Design review of the part built by this model. Coordinates are the model's own, in mm. Face numbers are marked on the shaded views. Coordinates: 2 decimals unless noted, no trailing zeros. Loops run counter-clockwise (first coordinate to the right, second up) from the corner with the lowest first, then second, coordinate; pieces in that order, holes last. Notation, with made-up numbers: M -31.75,24 L 12.25,24 A16 cw 12.25,48 Z; hole C 34,-32 d11. An arc over 180 degrees is marked long. One line per item, written item: value.
```python
from build123d import *

# Parameters (mm, degrees)
SKETCH1_R           = 20
BOSS_EXTRUDE1_DEPTH = 50
SHELL3_T            = -2
CUT_EXTRUDE1_DEPTH  = 50


with BuildPart() as part:
    # Sketch1 → Boss-Extrude1 (new body)
    with BuildSketch(Plane(origin=(0, 0, 0), x_dir=(1, 0, 0), z_dir=(0, 1, 0))):
        with Locations(Location((0, 0, 0), (0, 0, 270))):
            Circle(SKETCH1_R)
    extrude(amount=BOSS_EXTRUDE1_DEPTH)

    # Shell3
    shell3_openings = [part.faces().sort_by_distance(p)[0] for p in [
        (0, 50, 0),
    ]]
    offset(amount=SHELL3_T, openings=shell3_openings, kind=Kind.INTERSECTION)

    # Sketch2 → Cut-Extrude1 (cut)
    with BuildSketch(Plane(origin=(0, 2, 0), x_dir=(1, 0, 0), z_dir=(0, 1, 0))):
        with BuildLine():
            Line((-1, -16.970562748), (-1, 16.970562748))
            ThreePointArc((-1, 16.970562748), (-17, 0), (-1, -16.970562748))
        make_face()
        with BuildLine():
            ThreePointArc((17, 0), (12.369316877, 11.66190379), (1, 16.970562748))
            Line((1, 16.970562748), (1, -16.970562748))
            ThreePointArc((1, -16.970562748), (12.369316877, -11.66190379), (17, 0))
        make_face()
    extrude(amount=-CUT_EXTRUDE1_DEPTH, mode=Mode.SUBTRACT)


solid = part.part
```
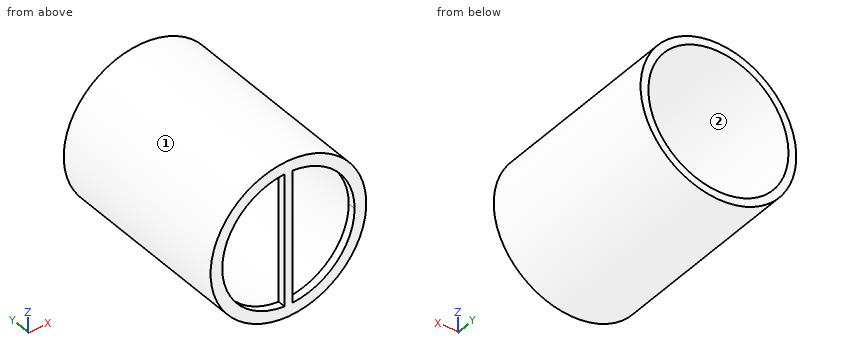
(1) We need section C-C on x = 0. State the section outline as (y, z) points.
Reply:
outline: M 0,-20 L 50,-20 L 50,-18 L 2,-18 L 2,18 L 50,18 L 50,20 L 0,20 Z
(2) We need section A-A on z = 1. State the section outline as (x, y) points, then the cut area to 3 significant figures.
Reply:
outline: M -19.97,0 L -16.97,0 L -16.97,2 L -17.97,2 L -17.97,50 L -19.97,50 Z; M -1,0 L 1,0 L 1,2 L -1,2 Z; M 16.97,0 L 19.97,0 L 19.97,50 L 17.97,50 L 17.97,2 L 16.97,2 Z
area: 208 mm2
(3) We need section B-B on x = 4.5. State the section outline as (y, z) points, then the cut area to 3 significant figures.
Reply:
outline: M 0,-19.49 L 50,-19.49 L 50,-17.43 L 2,-17.43 L 2,-16.39 L 0,-16.39 Z; M 0,16.39 L 2,16.39 L 2,17.43 L 50,17.43 L 50,19.49 L 0,19.49 Z
area: 210 mm2
(4) To check wall thickness, follow line 1 along X through (y, z) = (30, 0); line 2 along Z through (x, y) = (0.5, 15); line 3 along Z through (x, y) = (5.5, 23.5). State the ranges of each line that lie inside material, in increasing order. Write a range as [from, to].
Reply:
line 1: x = [-20, -18], [18, 20]
line 2: z = [-19.99, -17.99], [17.99, 19.99]
line 3: z = [-19.23, -17.14], [17.14, 19.23]
(5) Insertion check: pin 1 (4 mm diameter, centred on y = 24.5, z = -13.5, fed in from +X); pin 2 (1.6 mm diameter, centred on y = 1, z = -7.5, fed in from -X); pin 3 (1.5 mm diameter, centred on y = 38, z = -3.5, fed in from +X). Each pin has a flat end and moves straight along its axis. Give the tip position at first contact, or say it passes through.
Reply:
pin 1: stops at x = 16.36
pin 2: stops at x = -18.84
pin 3: stops at x = 19.81
(6) We need section D-D on y = 29.5. State the section outline as (x, z) points.
Reply:
outline: C 0,0 d40; hole C 0,0 d36
(7) Mouldability with a two-part tool opening along X and no side actions: class the marked faces 1 and 2 as released by +X, released by -X, zero draft, split by the parting line, or undercut.
Reply:
face 1: split by the parting line
face 2: undercut
